from build123d import *

# Parameters (mm, degrees)
BOSS_EXTRUDE1_DEPTH                                 = 9.5
CUT_EXTRUDE1_REACH                                  = 11.5
SKETCH2_R                                           = 12.8397
CSK_FOR_M2_COUNTERSUNK_FLAT_HEAD_SCREW1_D           = 2.4
CSK_FOR_M2_COUNTERSUNK_FLAT_HEAD_SCREW1_DEPTH       = 9.5
CSK_FOR_M2_COUNTERSUNK_FLAT_HEAD_SCREW1_CSINK_D     = 4.4
CSK_FOR_M2_COUNTERSUNK_FLAT_HEAD_SCREW1_CSINK_ANGLE = 90


with BuildPart() as part:
    # Sketch1 → Boss-Extrude1 (new body)
    with BuildSketch(Plane.XY):
        with BuildLine():
            Line((-16, -14.5), (16, -14.5))
            ThreePointArc((16, -14.5), (17.414213562, -13.914213562), (18, -12.5))
            Line((18, -12.5), (18, 14.5))
            Line((18, 14.5), (-18, 14.5))
            Line((-18, 14.5), (-18, -12.5))
            ThreePointArc((-18, -12.5), (-17.414213562, -13.914213562), (-16, -14.5))
        make_face()
    extrude(amount=BOSS_EXTRUDE1_DEPTH)

    # Sketch2 → Cut-Extrude1 (cut, up to next)
    with BuildSketch(Plane(origin=(0, 0, 9.5), x_dir=(0, 1, 0), z_dir=(0, 0, 1)), mode=Mode.PRIVATE) as cut_extrude1_sk1:
        Circle(SKETCH2_R)
    cut_extrude1_tool1 = extrude(cut_extrude1_sk1.sketch, amount=-CUT_EXTRUDE1_REACH, mode=Mode.PRIVATE) & part.part
    add(cut_extrude1_tool1.solids().sort_by_distance((0, 0, 9.5))[0], mode=Mode.SUBTRACT)

    # CSK for M2 Countersunk Flat Head Screw1
    with Locations(Plane.XY.offset(9.5)):
        with Locations((-14.7, 7), (14.7, 7)):
            CounterSinkHole(CSK_FOR_M2_COUNTERSUNK_FLAT_HEAD_SCREW1_D / 2, CSK_FOR_M2_COUNTERSUNK_FLAT_HEAD_SCREW1_CSINK_D / 2, depth=CSK_FOR_M2_COUNTERSUNK_FLAT_HEAD_SCREW1_DEPTH, counter_sink_angle=CSK_FOR_M2_COUNTERSUNK_FLAT_HEAD_SCREW1_CSINK_ANGLE)


solid = part.part
Check sheet for the modelled part. Datum: model origin and axes. Units: mm. Round coordinates to 2 decimals unless told otherwise and drop trailing zeros. Loops run counter-clockwise (first coordinate to the right, second up) from the corner with the lowest first, then second, coordinate; pieces in that order, holes last. Notation, with made-up numbers: M 77,67 L 131,67 A25 cw 131,85 Z; hole C 82.25,41.25 d1. An arc over 180 degrees is marked long. One line per item, written item: value.
(1) Release check for a two-part mould opening along X. For faces 1 (the face through (-15.35, 8.01, 4.19)), 2 (the face through (18, 1, 5)), 3 (the face through (-18, 1, 5)) record: +X half, -X half, draft (parallel to the pull), parting line (faces both ways), or undercut.
Computed values:
face 1: undercut
face 2: +X half
face 3: -X half
(2) Sectioned sample at C-C, the plane z = 5.25. Record the cut outline in (x, y).
Computed values:
outline: M -18,-12.5 A2 ccw -16,-14.5 L 16,-14.5 A2 ccw 18,-12.5 L 18,14.5 L -18,14.5 Z; hole C -14.7,7 d2.4; hole C 0,0 d25.68; hole C 14.7,7 d2.4
(3) Sectioned sample at D-D, the plane y = 7. Record the cut outline in (x, z).
Computed values:
outline: M -18,0 L -15.9,0 L -15.9,8.5 L -16.9,9.5 L -18,9.5 Z; M -13.5,0 L -10.76,0 L -10.76,9.5 L -12.5,9.5 L -13.5,8.5 Z; M 10.76,0 L 13.5,0 L 13.5,8.5 L 12.5,9.5 L 10.76,9.5 Z; M 15.9,0 L 18,0 L 18,9.5 L 16.9,9.5 L 15.9,8.5 Z
(4) Thickness scan on line 1 (Y direction, x = -14.7, z = 5); line 2 (Y direction, x = 0, z = 6); line 3 (X direction, y = 0, z = 4.75). Record the ranges inside material, lowest first.
Computed values:
line 1: y = -14.5 to 5.8, 8.2 to 14.5
line 2: y = -14.5 to -12.84, 12.84 to 14.5
line 3: x = -18 to -12.84, 12.84 to 18
(5) Sectioned sample at A-A, the plane x = 0. Record the cut outline in (y, z).
Computed values:
outline: M -14.5,0 L -12.84,0 L -12.84,9.5 L -14.5,9.5 Z; M 12.84,0 L 14.5,0 L 14.5,9.5 L 12.84,9.5 Z
(6) Sectioned sample at B-B, the plane y = 0. Record the cut outline in (x, z).
Computed values:
outline: M -18,0 L -12.84,0 L -12.84,9.5 L -18,9.5 Z; M 12.84,0 L 18,0 L 18,9.5 L 12.84,9.5 Z
